Autodesk Inventor part; units mm, degrees
ref_plane "YZ Plane" through (0, 0, 0) normal (1, 0, 0) x (0, 1, 0)
ref_plane "XZ Plane" through (0, 0, 0) normal (0, 1, 0) x (-1, 0, 0)
ref_plane "XY Plane" through (0, 0, 0) normal (0, 0, 1) x (1, 0, 0)
sketch "Sketch1" plane through (0, 0, 0) normal (0, 1, 0) x (-1, 0, 0)
  line L0 (28.6465, 75.6443) -> (-1.3535, 75.6443)
  line L1 (-1.3535, 75.6443) -> (-1.3535, -4.3557)
  line L2 (-1.3535, -4.3557) -> (28.6465, -4.3557)
  line L3 (28.6465, -4.3557) -> (28.6465, 75.6443)
  point P0 (0, 0)
  dimension "d0" = 30
  dimension "d1" = 80
extrude "Extrusion1" add sketch "Sketch1" along normal blind 5
sketch "Sketch2" plane through (0, 5, 0) normal (0, 1, 0) x (1, 0, 0)
  line L0 (1.3535, -75.6443) -> (1.3535, 4.3557)
  line L1 (-28.6465, -75.6443) -> (1.3535, -75.6443)
  line L2 (1.3535, -75.6443) -> (1.3535, -60.6443)
  line L3 (1.3535, -60.6443) -> (-28.6465, -60.6443)
  line L4 (-28.6465, -60.6443) -> (-28.6465, -75.6443)
  line L5 (-28.6465, 4.3557) -> (1.3535, 4.3557)
  line L6 (1.3535, 4.3557) -> (1.3535, -10.6443)
  line L7 (1.3535, -10.6443) -> (-28.6465, -10.6443)
  line L8 (-28.6465, -10.6443) -> (-28.6465, 4.3557)
  line L9 (-28.6465, -60.6443) -> (1.3535, -60.6443)
  line L10 (1.3535, -60.6443) -> (1.3535, -10.6443)
  line L11 (1.3535, -10.6443) -> (-28.6465, -10.6443)
  line L12 (-28.6465, -10.6443) -> (-28.6465, -60.6443)
  point P0 (0, 0)
  dimension "d4" = 15
  dimension "d5" = 15
extrude "Extrusion2" add sketch "Sketch2" along normal blind 15 contours L3 L12 L7 L0
sketch "Sketch3" plane through (0, 20, 0) normal (0, 1, 0) x (1, 0, 0)
  line L0 (1.3535, -60.6443) -> (-28.6465, -60.6443)
  line L1 (-13.6465, -60.6443) -> (-13.6465, -10.6443)
  line L2 (1.3535, -10.6443) -> (-28.6465, -10.6443)
  line L3 (-28.6465, 4.3557) -> (-28.6465, -75.6443)
  line L4 (-28.6465, -35.6443) -> (1.3535, -35.6443)
  line L5 (1.3535, -75.6443) -> (1.3535, 4.3557)
  line L6 (-13.6465, -60.6443) -> (-13.6465, -36.1443)
  line L7 (-13.6465, -60.6443) -> (-13.6465, -48.1443)
  circle A0 centre (-13.6465, -48.1443) radius 7.5
  circle A1 centre (-13.6465, -23.1443) radius 7.5
  point P0 (0, 0)
  dimension "d8" = 50
  dimension "d9" = 24.5
  dimension "d10" = 12.5
  dimension "d11" = 15
extrude "Extrusion4" cut sketch "Sketch3" against normal blind 8 contours A0 L1 | L1 A0 | A1 L1 | L1 A1
properties part number "sonar"
Can you work these out from the model? Positions are in its coordinate system, mm. A direction names the side the tool comes from. Round coordinates to 2 decimals unless told otherwise and drop trailing zeros. Loops run counter-clockwise (first coordinate to the right, second up) from the corner with the lowest first, then second, coordinate; pieces in that order, holes last. Notation, with made-up numbers: (-36.75, 52.5) - (-7.75, 52.5) arc R24 ccw to (-7.75, 70.5) - close; hole circle Ø3 at (28.5, -32.75). An arc over 180 degrees is marked (long way). Use CSV: the item, a comma, the result in double quotes. Start each with the question number.
1) For faces 5 (the flat face through (-13, 5, 3)), 6 (the flat face through (-13, 2, -4.356)), 7 (the flat face through (-14, 12, 23)), 8 (the flat face through (-13, 5, 68)), which set-ups out of +Z, -Z, +X, -X, +Y, -Y let a thin tool reach every point of the face, with its end or its side?
2) If we section it at C-C on y = 17.25: Write out the boundary of the cut face in (x, z).
3) For pin 1 Ø4.5 at (x, z) = (-10, 70) entering from +Y; pin 2 Ø4 at (x, y) = (-11, 16) entering from -Z; pin 3 Ø4.5 at (x, y) = (-6.5, 15) entering from +Z, each with a flat end and sliding along its axis, tell me the tip position at first contact or that it passes through.
4) If we section it at A-A on x = -2.5: Write out the boundary of the cut face in (y, z).
5) We'd pull the mould along X, two halves only. Please class faces 1 (the flat face through (-28.646, 8, 35)), 2 (the flat face through (-14, 20, 35)), 3 (the flat face through (-14, 12, 48)), 4 (the cylindrical face through (-15.272, 16.056, 30.466)): released by +X, released by -X, zero draft, split by the parting line, or undercut.
6) If we section it at B-B on z = 53: Write out the boundary of the cut face in (x, y), plus the area to 3 significant figures.
7) If we section it at D-D on x = -9.5: Write out the boundary of the cut face in (y, z), plus the area to 3 significant figures.
8) Please list where these lines run through material, in increasing order: probe 1 along Z at (x, y) = (-9, 13); probe 2 along Z at (x, y) = (-24.25, 10); probe 3 along Y at (x, z) = (-3.5, 2). Write a range as [from, to].
Geometry results:
1,face 5,"-Z, +X, -X, +Y"
1,face 6,"-Z, +X, -X, +Y, -Y"
1,face 7,"+Y"
1,face 8,"+Z, +X, -X, +Y"
2,outline,"(-28.65, 10.64) - (1.35, 10.64) - (1.35, 60.64) - (-28.65, 60.64) - close; hole circle Ø15 at (-13.65, 23.14); hole circle Ø15 at (-13.65, 48.14)"
3,pin 1,"stops at y = 5"
3,pin 2,"stops at z = 10.64"
3,pin 3,"stops at z = 60.64"
4,outline,"(0, -4.36) - (5, -4.36) - (5, 10.64) - (20, 10.64) - (20, 60.64) - (5, 60.64) - (5, 75.64) - (0, 75.64) - close"
5,face 1,"released by -X"
5,face 2,"zero draft"
5,face 3,"undercut"
5,face 4,"undercut"
6,outline,"(-28.65, 0) - (1.35, 0) - (1.35, 20) - (-7.93, 20) - (-7.93, 12) - (-19.36, 12) - (-19.36, 20) - (-28.65, 20) - close"
6,area,"509 mm2"
7,outline,"(0, -4.36) - (5, -4.36) - (5, 10.64) - (20, 10.64) - (20, 16.89) - (12, 16.89) - (12, 29.39) - (20, 29.39) - (20, 41.89) - (12, 41.89) - (12, 54.39) - (20, 54.39) - (20, 60.64) - (5, 60.64) - (5, 75.64) - (0, 75.64) - close"
7,area,"950 mm2"
8,probe 1,"z = [10.64, 17.26], [29.03, 42.26], [54.03, 60.64]"
8,probe 2,"z = [10.64, 60.64]"
8,probe 3,"y = [0, 5]"
